Build history of the part. All positions in model axes, mm. A direction names the side the tool comes from. Round coordinates to 2 decimals unless told otherwise and drop trailing zeros. Loops run counter-clockwise (first coordinate to the right, second up) from the corner with the lowest first, then second, coordinate; pieces in that order, holes last. Notation, with made-up numbers: (-22, 38) - (31, 38) arc R31 ccw to (31, 65) - close; hole circle Ø10 at (74, 26). An arc over 180 degrees is marked (long way). Use a Markdown table: item, result.
from build123d import *

# Parameters (mm, degrees)
SKETCH3_W            = 40
SKETCH3_H            = 34
SKETCH3_R            = 0.25
SKETCH3_R_2          = 0.5
BOSS_EXTRUDE2_DEPTH  = 2
SKETCH4_R            = 6
BOSS_EXTRUDE3_DEPTH  = 2
SKETCH5_R            = 11.899793619
BOSS_EXTRUDE4_DEPTH  = 1
SKETCH7_R            = 11.354972543
SKETCH7_R_2          = 6
CUT_EXTRUDE1_DEPTH   = 2
BOSS_EXTRUDE5_DEPTH  = 24
SKETCH11_W           = 16
SKETCH11_H           = 22
CUT_EXTRUDE2_DEPTH   = 10
SKETCH12_R           = 2.5
BOSS_EXTRUDE6_DEPTH  = 24
CUT_EXTRUDE3_DEPTH   = 26
FILLET3_R            = 8
FILLET4_R            = 8
FILLET5_R            = 8
FILLET6_R            = 8
SKETCH16_W           = 40.5
SKETCH16_H           = 34.5
BOSS_EXTRUDE12_DEPTH = 4
SKETCH21_R           = 1.5
CUT_EXTRUDE10_DEPTH  = 8
FILLET13_R           = 0.5
FILLET15_R           = 8


with BuildPart() as part:
    # Sketch3 → Boss-Extrude2 (new body)
    with BuildSketch(Plane.XY):
        with Locations((67.033183219, 114.752969631)):
            Rectangle(SKETCH3_W, SKETCH3_H)
        with Locations((82.033183219, 126.752969631)):
            Circle(SKETCH3_R, mode=Mode.SUBTRACT)
        with Locations((52.033183219, 126.752969631)):
            Circle(SKETCH3_R_2, mode=Mode.SUBTRACT)
        with Locations((52.033183219, 102.752969631)):
            Circle(SKETCH3_R, mode=Mode.SUBTRACT)
        with Locations((82.033183219, 102.752969631)):
            Circle(SKETCH3_R_2, mode=Mode.SUBTRACT)
    extrude(amount=BOSS_EXTRUDE2_DEPTH)

    # Sketch4 → Boss-Extrude3 (add)
    with BuildSketch(Plane.XY.offset(2)):
        with Locations((67.537199027, 114.923254134)):
            Circle(SKETCH4_R)
    extrude(amount=BOSS_EXTRUDE3_DEPTH)

    # Sketch5 → Boss-Extrude4 (add)
    with BuildSketch(Plane.XY.offset(2)):
        with Locations((67.537199027, 114.923254134)):
            Circle(SKETCH5_R)
    extrude(amount=BOSS_EXTRUDE4_DEPTH)

    # Sketch7 → Cut-Extrude1 (cut)
    with BuildSketch(Plane.XY.offset(4)):
        with Locations((67.537199027, 114.923254134)):
            Circle(SKETCH7_R)
        with Locations((67.537199027, 114.923254134)):
            Circle(SKETCH7_R_2, mode=Mode.SUBTRACT)
    extrude(amount=-CUT_EXTRUDE1_DEPTH, mode=Mode.SUBTRACT)

    # Sketch10 → Boss-Extrude5 (add)
    with BuildSketch(Plane(origin=(0, 103, 0), x_dir=(1, 0, 0), z_dir=(0, 1, 0))):
        Polygon((66.720095213, -1.747898749), (56.543730993, -18.18677206), (56.543730993, -2.18677206), align=None)
    extrude(amount=BOSS_EXTRUDE5_DEPTH)

    # Sketch11 → Cut-Extrude2 (cut)
    with BuildSketch(Plane.ZY.offset(-56.543730993)):
        with Locations((10.18677206, 115)):
            Rectangle(SKETCH11_W, SKETCH11_H)
    extrude(amount=-CUT_EXTRUDE2_DEPTH, mode=Mode.SUBTRACT)

    # Sketch12 → Boss-Extrude6 (add)
    with BuildSketch(Plane.XZ.offset(-103)):
        with Locations((57.268401618, 15.213410807)):
            Circle(SKETCH12_R)
    extrude(amount=-BOSS_EXTRUDE6_DEPTH)

    # Sketch14 → Cut-Extrude3 (cut)
    with BuildSketch(Plane(origin=(0, 127, 0), x_dir=(1, 0, 0), z_dir=(0, 1, 0))):
        Polygon((56.543730993, -17.606077203), (56.543730993, -18.18677206), (56.857779916, -17.679458215), align=None)
    extrude(amount=-CUT_EXTRUDE3_DEPTH, mode=Mode.SUBTRACT)

    # Fillet3
    fillet3_edges = [part.edges().sort_by_distance(p)[0] for p in [
        (87.033183219, 131.752969631, 1),
    ]]
    fillet(fillet3_edges, radius=FILLET3_R)

    # Fillet4
    fillet4_edges = [part.edges().sort_by_distance(p)[0] for p in [
        (87.033183219, 97.752969631, 1),
    ]]
    fillet(fillet4_edges, radius=FILLET4_R)

    # Fillet5
    fillet5_edges = [part.edges().sort_by_distance(p)[0] for p in [
        (47.033183219, 131.752969631, 1),
    ]]
    fillet(fillet5_edges, radius=FILLET5_R)

    # Fillet6
    fillet6_edges = [part.edges().sort_by_distance(p)[0] for p in [
        (47.033183219, 97.752969631, 1),
    ]]
    fillet(fillet6_edges, radius=FILLET6_R)

    # Sketch16 → Boss-Extrude12 (add)
    with BuildSketch(Plane(origin=(0, 0, 0), x_dir=(-1, 0, 0), z_dir=(0, 0, -1))):
        with Locations((-67.069775125, 114.708699914)):
            Rectangle(SKETCH16_W, SKETCH16_H)
    extrude(amount=BOSS_EXTRUDE12_DEPTH)

    # Sketch21 → Cut-Extrude10 (cut)
    with BuildSketch(Plane(origin=(0, 0, -4), x_dir=(-1, 0, 0), z_dir=(0, 0, -1))):
        with Locations((-82.069775125, 126.708699914)):
            Circle(SKETCH21_R)
        with Locations((-52.069775125, 126.708699914)):
            Circle(SKETCH21_R)
        with Locations((-52.069775125, 102.708699914)):
            Circle(SKETCH21_R)
        with Locations((-82.069775125, 102.708699914)):
            Circle(SKETCH21_R)
    extrude(amount=-CUT_EXTRUDE10_DEPTH, mode=Mode.SUBTRACT)

    # Fillet13
    fillet13_edges = [part.edges().sort_by_distance(p)[0] for p in [
        (67.033183219, 131.752969631, 2),
        (84.690037469, 129.409823881, 2),
        (87.033183219, 114.752969631, 2),
        (84.690037469, 100.096115382, 2),
        (47.033183219, 114.752969631, 2),
        (49.37632897, 129.409823881, 2),
        (67.033183219, 97.752969631, 2),
        (49.37632897, 100.096115382, 2),
    ]]
    fillet(fillet13_edges, radius=FILLET13_R)

    # Fillet15
    fillet15_edges = [part.edges().sort_by_distance(p)[0] for p in [
        (87.319775125, 131.958699914, -2),
        (87.319775125, 97.458699914, -2),
        (46.819775125, 97.458699914, -2),
        (46.819775125, 131.958699914, -2),
    ]]
    fillet(fillet15_edges, radius=FILLET15_R)


solid = part.part
Q1. Cut at C-C, the plane x = 71.5. List the corners of the cut face in (y, z).
Results found:
| item | result |
|---|---|
| outline | (97.46, -4) - (131.96, -4) - (131.96, 0) - (131.75, 0) - (131.75, 1.5) arc R0.5 ccw to (131.25, 2) - (126.14, 2) - (126.14, 3) - (125.56, 3) - (125.56, 2) - (119.43, 2) - (119.43, 4) - (110.42, 4) - (110.42, 2) - (104.28, 2) - (104.28, 3) - (103.7, 3) - (103.7, 2) - (98.25, 2) arc R0.5 ccw to (97.75, 1.5) - (97.75, 0) - (97.46, 0) - close |
Q2. Which spindle directions (+Z, -Z, +X, -X, +Y, -Y) get a long thin tool onto all of the face, cutting with end or side? Do faces 1 (the face through (57, 115, 2)), 2 (the face through (87.033, 115, 1)), 3 (the face through (47.033, 115, 1)), 4 (the face through (67, 131.753, 1)). Say none if no direction does.
Results found:
| item | result |
|---|---|
| face 1 | none |
| face 2 | +Z, +X, +Y, -Y |
| face 3 | +Z, -X, +Y, -Y |
| face 4 | +Z, +X, -X, +Y |
Q3. Cut at D-D, the plane z = -2.5. List the corners of the cut face in (x, y).
Results found:
| item | result |
|---|---|
| outline | (46.82, 105.46) arc R8 ccw to (54.82, 97.46) - (79.32, 97.46) arc R8 ccw to (87.32, 105.46) - (87.32, 123.96) arc R8 ccw to (79.32, 131.96) - (54.82, 131.96) arc R8 ccw to (46.82, 123.96) - close; hole circle Ø3 at (52.07, 102.71); hole circle Ø3 at (52.07, 126.71); hole circle Ø3 at (82.07, 102.71); hole circle Ø3 at (82.07, 126.71) |
Q4. Cut at A-A, the plane z = 10.25. List the corners of the cut face in (x, y), plus the area to 3 significant figures.
Results found:
| item | result |
|---|---|
| outline | (56.54, 103) - (61.46, 103) - (61.46, 104) - (56.54, 104) - close; (56.54, 126) - (61.46, 126) - (61.46, 127) - (56.54, 127) - close |
| area | 9.83 mm2 |
Q5. Cut at B-B, the plane x = 58.5. List the corners of the cut face in (y, z), plus the area to 3 significant figures.
Results found:
| item | result |
|---|---|
| outline | (97.46, -4) - (131.96, -4) - (131.96, 0) - (131.75, 0) - (131.75, 1.5) arc R0.5 ccw to (131.25, 2) - (122.66, 2) - (122.66, 2.1) - (127, 2.1) - (127, 17.39) - (103, 17.39) - (103, 2.1) - (107.18, 2.1) - (107.18, 2) - (98.25, 2) arc R0.5 ccw to (97.75, 1.5) - (97.75, 0) - (97.46, 0) - close; hole (104, 2.19) - (126, 2.19) - (126, 13.04) - (104, 13.04) - close; hole (108.05, 2) - (121.8, 2) - (121.8, 2.1) - (108.05, 2.1) - close |
| area | 334 mm2 |
Q6. Pull direction Z, two halves, no side cores. Call faces 5 (the face through (67, 115, -4)), 6 (the face through (67, 97.753, 1)), 7 (the face through (56, 115, 3)): pulls with the +Z half, pulls with the -Z half, needs draft (parallel to the pull), parting line crosses it, or undercut.
Results found:
| item | result |
|---|---|
| face 5 | pulls with the -Z half |
| face 6 | needs draft |
| face 7 | undercut |
Q7. Drop flat-ended pins along their axis: pin 1 (0.8 mm diameter, centred on y = 126.5, z = 7, fed in from -X); pin 2 (2.5 mm diameter, centred on x = 52.07, y = 102.71, fed in from +Z); pin 3 (0.9 mm diameter, centred on y = 114, z = 2.5, fed in from -X); pin 4 (4 mm diameter, centred on x = 74, y = 105.5, fed in from +Z). Give the stop position or say it passes through.
Results found:
| item | result |
|---|---|
| pin 1 | stops at x = 56.54 |
| pin 2 | passes through |
| pin 3 | stops at x = 55.65 |
| pin 4 | stops at z = 3 |
Q8. Probe line 1 (Y direction, x = 81.5, z = -1); line 2 (Y direction, x = 64.5, z = 3); line 3 (Z direction, x = 52, y = 118). List the from-to ranges inside material, lowest first.
Results found:
| item | result |
|---|---|
| line 1 | y = 97.76 to 101.32, 104.1 to 125.32, 128.1 to 131.66 |
| line 2 | y = 103 to 104, 126 to 127 |
| line 3 | z = -4 to 2 |
